Verification items for the finished model (mm, model axes). Give positions to 0.01 mm unless a question says otherwise; leave off trailing zeros. Order: outer loops, then holes, each group sorted by start corner. A loop starts at its lowest first (then second) coordinate and runs counter-clockwise, first axis right, second up.
(1) Gauge pin test, flat ends, axial feed: pin 1 (1.5 mm diameter, centred on x = 1, y = 2, fed in from +Z); pin 2 (2.5 mm diameter, centred on x = 0, y = -7.5, fed in from -Z). Record the tip position at first contact, or that the pin passes through.
(2) Scan lines: L1, parallel to Y at x = 0, z = 0.8; L2, parallel to Y at x = 1, z = 0.55; L3, parallel to Z at x = -2.5, y = -3. Record each from-to range of solid material in increasing order.
(3) Sectioned sample at C-C on z = 1. Record the cut outline in (x, y), plus the area to 3 significant figures.
(4) Sectioned sample at B-B on x = 0.25. Record the cut outline in (y, z).
(5) Mould release check, pull along Y, two halves, no side actions. Record for faces 1 (the face through (3.5, 0, 1)), 2 (the face through (0, -11, 1)), 3 (the face through (-0.37, -5.84, 0.59)), 4 (the face through (-0.759, 10.917, 1.382)): pulls with the +Y half, pulls with the -Y half, needs draft (parallel to the pull), parting line crosses it, or undercut.
(6) Sectioned sample at A-A on y = 6.75. Record the cut outline in (x, z) (3 decimals).
(7) Sectioned sample at D-D on x = 2. Record the cut outline in (y, z).
Autodesk Inventor part; units mm, degrees
ref_plane "YZ Plane" through (0, 0, 0) normal (1, 0, 0) x (0, 1, 0)
ref_plane "XZ Plane" through (0, 0, 0) normal (0, 1, 0) x (-1, 0, 0)
ref_plane "XY Plane" through (0, 0, 0) normal (0, 0, 1) x (1, 0, 0)
sketch "Náčrt1" plane through (0, 0, 0) normal (0, 0, 1) x (1, 0, 0)
  line L0 (0, 7.5) -> (0, -7.5) construction
  line L1 (-3.5, 7.5) -> (-3.5, -7.5)
  line L2 (3.5, -7.5) -> (3.5, 7.5)
  arc A0 (3.5, 7.5) -> (-3.5, 7.5) centre (0, 7.5) ccw
  arc A1 (-3.5, -7.5) -> (3.5, -7.5) centre (0, -7.5) ccw
  circle A2 centre (0, 7.5) radius 1.7
  circle A3 centre (0, -7.5) radius 1.7
  circle A4 centre (0, 7.5) radius 3.5
  point P0 (0, 0)
  point P1 (0, 0)
  point P2 (3.5, 7.5)
  dimension "d0" = 15
  dimension "d1" = 3.5
  dimension "d2" = 3.4
extrude "Vysunutí1" add sketch "Náčrt1" along normal blind 1.2
extrude "Vysunutí2" add sketch "Náčrt1" along normal blind 2.5 contours A0 A4
sketch "Náčrt4" plane through (3.5, -7.5, 0) normal (1, 0, 0) x (0, 0, -1)
  line L0 (-2.5, 13.3) -> (-2.5, 16.7)
  line L1 (-1.2, -1.7) -> (-1.2, 1.7)
  line L2 (-2.5, 15) -> (-1.2, 0)
  line L3 (-2.5, 18.5) -> (-2.5, 11.5)
  line L4 (0, 15) -> (0, 15)
  line L5 (0, 15) -> (-1.2, 15)
  line L6 (-1.2, 15) -> (-1.2, 15)
  line L7 (0, 15) -> (-1.2, 15)
  line L8 (-1.2, 11.5) -> (-2.5, 11.5)
  line L9 (-2.5, 15) -> (-2.8033, 18.5)
  line L10 (-2.5, 18.5) -> (-2.8033, 18.5)
  point P0 (0, 7.5)
  point P1 (-2.1967, 11.5)
extrude "Vysunutí3" cut sketch "Náčrt4" against normal through all contours L0 L2 L8 L3
extrude "Vysunutí4" add sketch "Náčrt4" against normal up to surface (7 mm away) contours L9 L10 L3 L0
sketch "Náčrt5" plane through (0, 0, 0) normal (0, 0, -1) x (-1, 0, 0)
  circle A0 centre (0, 7.5) radius 1.7
  circle A1 centre (0, -7.5) radius 1.7
  line L0 (-3.5, -7.5) -> (-3.5, 7.5)
  arc A2 (-3.5, -7.5) -> (3.5, -7.5) centre (0, -7.5) ccw
  line L1 (3.5, 7.5) -> (3.5, -7.5)
  arc A3 (3.5, 7.5) -> (-3.5, 7.5) centre (0, 7.5) ccw
  arc A4 (1.7, 7.5) -> (-1.7, 7.5) centre (0, 7.5) ccw
  line L2 (-1.7, 7.5) -> (1.7, 7.5)
  arc A5 (3.5, 7.5) -> (0, 11) centre (0, 7.5) ccw
  line L3 (3.5, 11) -> (3.5, 7.5)
  line L4 (0, 11) -> (3.5, 11)
  arc A6 (0, 11) -> (-3.5, 7.5) centre (0, 7.5) ccw
  line L5 (-3.5, 11) -> (0, 11)
  line L6 (-3.5, 7.5) -> (-3.5, 11)
  point P0 (0, 0)
  point P1 (3.5, 7.5)
  point P2 (0, 11)
  point P3 (0, 11)
  point P4 (0, 11)
  point P5 (-3.5, 7.5)
  point P6 (-1.7, 7.5)
  point P7 (1.7, 7.5)
extrude "Vysunutí5" cut sketch "Náčrt5" against normal through all contours L2 A0 | L6 L5 A3 | L4 L3 A3 picked at (0.5018, 7.7633)
properties part number "back qre flex holder"
Ans:
1. pin 1: stops at z = 1.2
1. pin 2: passes through
2. L1: y = -11 to -9.2, -5.8 to 5.8, 9.2 to 11
2. L2: y = -10.85 to -8.87, -6.13 to 6.13, 8.87 to 10.85
2. L3: z = 0 to 1.2
3. outline: (-3.5, -7.5) arc R3.5 ccw to (3.5, -7.5) - (3.5, 7.5) arc R3.5 ccw to (-3.5, 7.5) - close; hole circle Ø3.4 at (0, -7.5); hole circle Ø3.4 at (0, 7.5)
3. area: 125 mm2
4. outline: (-10.99, 0) - (-9.18, 0) - (-9.18, 1.2) - (-10.99, 1.2) - close; (-5.82, 0) - (5.82, 0) - (5.82, 2.35) - (4.01, 2.2) - (4.01, 1.2) - (-5.82, 1.2) - close; (9.18, 0) - (10.99, 0) - (10.99, 2.8) - (9.18, 2.65) - close
5. face 1: needs draft
5. face 2: pulls with the -Y half
5. face 3: undercut
5. face 4: parting line crosses it
6. outline: (-3.5, 0) - (-1.526, 0) - (-1.526, 2.435) - (-3.419, 2.435) - (-3.419, 1.2) - (-3.5, 1.2) - close; (1.526, 0) - (3.5, 0) - (3.5, 1.2) - (3.419, 1.2) - (3.419, 2.435) - (1.526, 2.435) - close
7. outline: (-10.37, 0) - (10.37, 0) - (10.37, 2.75) - (7.5, 2.5) - (4.63, 2.25) - (4.63, 1.2) - (-10.37, 1.2) - close
